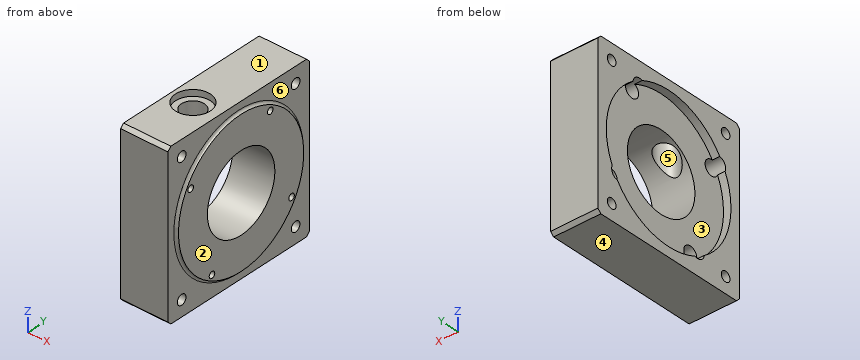
from build123d import *

# Parameters (mm, degrees)
SALIENTE_EXTRUIR1_DEPTH            = 38
TALADRO_DE_MARGEN_PARA_M1001_D     = 114.5
TALADRO_DE_MARGEN_PARA_M1001_DEPTH = 6
CROQUIS9_W                         = 34
CROQUIS9_H                         = 31
TALADRO_DE_MARGEN_PARA_M71_D       = 8


# Read off the part's stored shape, not the designer's step: Refrentado para perno con cabeza hexagonal de M161
with BuildPart() as part:
    # Croquis1 → Saliente-Extruir1 (new body)
    with BuildSketch(Plane(origin=(-94.5, 0, 0), x_dir=(0, -1, 0), z_dir=(-1, 0, 0))):
        with BuildLine():
            Line((62.24949799, 65), (-62.24949799, 65))
            ThreePointArc((-62.24949799, 65), (-63.639610307, 63.639610307), (-65, 62.24949799))
            Line((-65, 62.24949799), (-65, -62.24949799))
            ThreePointArc((-65, -62.24949799), (-63.639610307, -63.639610307), (-62.24949799, -65))
            Line((-62.24949799, -65), (62.24949799, -65))
            ThreePointArc((62.24949799, -65), (63.639610307, -63.639610307), (65, -62.24949799))
            Line((65, -62.24949799), (65, 62.24949799))
            ThreePointArc((65, 62.24949799), (63.639610307, 63.639610307), (62.24949799, 65))
        make_face()
    extrude(amount=-SALIENTE_EXTRUIR1_DEPTH)

    # Taladro de margen para M1001
    with Locations(Plane.ZY.offset(94.5)):
        with Locations((0, 0)):
            Hole(TALADRO_DE_MARGEN_PARA_M1001_D / 2, depth=TALADRO_DE_MARGEN_PARA_M1001_DEPTH)

    # Croquis4 → Revolución1 (revolve)
    with BuildSketch(Plane(origin=(0, 0, 0), x_dir=(-1, 0, 0), z_dir=(0, 0, -1)), mode=Mode.PRIVATE) as revoluci_n1_sk:
        with BuildLine():
            Line((54.5, 57.5), (54.5, 0))
            Line((54.5, 0), (56.5, 0))
            Line((56.5, 0), (56.5, 59.5))
            ThreePointArc((56.5, 59.5), (55.914213562, 58.085786438), (54.5, 57.5))
        make_face()
    revolve(revoluci_n1_sk.sketch.rotate(Axis((-54.499975, 0, 0), (-1, 0, 0)), 270), axis=Axis((-54.499975, 0, 0), (-1, 0, 0)))

    # Croquis5 → Cortar-Revolución1 (revolve, cut)
    with BuildSketch(Plane(origin=(0, 0, 46.3323591), x_dir=(-1, 0, 0), z_dir=(0, 0, -1)), mode=Mode.PRIVATE) as cortar_revoluci_n1_sk:
        Polygon((54.5, 29.3), (54.5, 26.75), (94.5, 26.75), (94.5, 32.75), (63.5, 32.75), (63.5, 29.3), align=None)
    revolve(cortar_revoluci_n1_sk.sketch.rotate(Axis((-54.5, 26.75, 46.3323591), (-1, 0, 0)), 270), axis=Axis((-54.5, 26.75, 46.3323591), (-1, 0, 0)), mode=Mode.SUBTRACT)

    # Croquis6 → Cortar-Revolución2 (revolve, cut)
    with BuildSketch(Plane(origin=(0, 0, -26.75), x_dir=(-1, 0, 0), z_dir=(0, 0, -1)), mode=Mode.PRIVATE) as cortar_revoluci_n2_sk:
        Polygon((54.5, 48.8823591), (54.5, 46.3323591), (94.5, 46.3323591), (94.5, 52.3323591), (63.5, 52.3323591), (63.5, 48.8823591), align=None)
    revolve(cortar_revoluci_n2_sk.sketch.rotate(Axis((-54.5, 46.3323591, -26.75), (-1, 0, 0)), 270), axis=Axis((-54.5, 46.3323591, -26.75), (-1, 0, 0)), mode=Mode.SUBTRACT)

    # Croquis7 → Cortar-Revolución3 (revolve, cut)
    with BuildSketch(Plane(origin=(0, 0, -46.3323591), x_dir=(-1, 0, 0), z_dir=(0, 0, -1)), mode=Mode.PRIVATE) as cortar_revoluci_n3_sk:
        Polygon((54.5, -24.2), (54.5, -26.75), (94.5, -26.75), (94.5, -20.75), (63.5, -20.75), (63.5, -24.2), align=None)
    revolve(cortar_revoluci_n3_sk.sketch.rotate(Axis((-54.5, -26.75, -46.3323591), (-1, 0, 0)), 270), axis=Axis((-54.5, -26.75, -46.3323591), (-1, 0, 0)), mode=Mode.SUBTRACT)

    # Croquis8 → Cortar-Revolución4 (revolve, cut)
    with BuildSketch(Plane(origin=(0, 0, 26.75), x_dir=(-1, 0, 0), z_dir=(0, 0, -1)), mode=Mode.PRIVATE) as cortar_revoluci_n4_sk:
        Polygon((54.5, -43.7823591), (54.5, -46.3323591), (94.5, -46.3323591), (94.5, -40.3323591), (63.5, -40.3323591), (63.5, -43.7823591), align=None)
    revolve(cortar_revoluci_n4_sk.sketch.rotate(Axis((-54.5, -46.3323591, 26.75), (-1, 0, 0)), 270), axis=Axis((-54.5, -46.3323591, 26.75), (-1, 0, 0)), mode=Mode.SUBTRACT)

    # Croquis9 → Cortar-Revolución5 (revolve, cut)
    with BuildSketch(Plane.XY, mode=Mode.PRIVATE) as cortar_revoluci_n5_sk:
        with Locations((-71.5, 15.5)):
            Rectangle(CROQUIS9_W, CROQUIS9_H)
    revolve(cortar_revoluci_n5_sk.sketch.rotate(Axis((-88.5, 0, 0), (1, 0, 0)), 270), axis=Axis((-88.5, 0, 0), (1, 0, 0)), mode=Mode.SUBTRACT)

    # Refrentado para perno con cabeza hex 2 → Refrentado para perno con cabeza hexagonal de M161 (revolve, cut)
    with BuildSketch(Plane(origin=(-77.5, -18, 0), x_dir=(1, 0, 0), z_dir=(0, -1, 0))):
        Polygon((0, 14.891701752), (9.188095, 14.891701752), (9.188095, 60), (14, 60), (14, 65), (0, 65), align=None)
    revolve(axis=Axis((-77.5, -18, 0), (0, 0, 1)), mode=Mode.SUBTRACT)

    # Taladro de margen para M71 (through all)
    with Locations(Plane.ZY.offset(94.5)):
        with Locations((-52.325901808, 52.325901808), (52.325901808, 52.325901808), (52.325901808, -52.325901808), (-52.325901808, -52.325901808)):
            Hole(TALADRO_DE_MARGEN_PARA_M71_D / 2)


solid = part.part
Verification items for the finished model (mm, model axes). Face numbers are marked on the shaded views. A direction names the side the tool comes from. Coordinates: 2 decimals unless noted, no trailing zeros. Order: outer loops, then holes, each group sorted by start corner. A loop starts at its lowest first (then second) coordinate and runs counter-clockwise, first axis right, second up. Notation, with made-up numbers: M 66.5,73 L 103.5,73 A26 ccw 103.5,91 Z; hole C -39,43 d2. An arc over 180 degrees is marked long. One line per item, written item: value. Start each with the question number.
Item 1: Depth check by flat-ended pin: P1, Ø6, axis at y = 22.5, z = 15, coming from the +X side; P2, Ø3.5, axis at y = -27, z = -44, coming from the -X side; P3, Ø9, axis at y = -52.33, z = 52.33, coming from the +X side; P4, Ø9.5, axis at y = -43.5, z = 26.5, coming from the -X side. Enter the tip coordinate at first touch or a pass-through.
Item 2: Sectioned sample at C-C on x = -77. Give the number of separate pieces and of enclosed holes in the cut face, then the cut area to 3 significant figures.
Item 3: Access from +Z, -Z, +X, -X, +Y, -Y to the whole of each face (thin tool, end or side, straight path). Record for the marked faces 4, 5 and 6.
Item 4: Sectioned sample at A-A on y = 0. Record the cut outline in (x, z).
Item 5: Thickness scan on probe 1 along Y at (x, z) = (-66, 52.5); probe 2 along Z at (x, y) = (-61, -26); probe 3 along Y at (x, z) = (-57.5, -26.75). Record the ranges inside material, lowest first.
Item 6: Mould release check, pull along Z, two halves, no side actions. Record for the marked faces 1, 2 and 3: pulls with the +Z half, pulls with the -Z half, needs draft (parallel to the pull), parting line crosses it, or undercut.
Calculated:
1. P1: through
1. P2: x = -63.5
1. P3: x = -56.5
1. P4: x = -88.5
2. separate pieces: 1
2. enclosed holes: 8
2. area: 12,400 mm^2
3. face 4: -Z, +X, -X, +Y, -Y
3. face 5: +Z
3. face 6: +X
4. outline: M -94.5,-65 L -56.5,-65 L -56.5,-59.5 A2 cw -54.5,-57.5 L -54.5,-31 L -88.5,-31 L -88.5,-57.25 L -94.5,-57.25 Z; M -94.5,57.25 L -88.5,57.25 L -88.5,31 L -54.5,31 L -54.5,57.5 A2 cw -56.5,59.5 L -56.5,65 L -94.5,65 Z
5. probe 1: -65 to -56.32, -48.33 to 48.33, 56.32 to 65
5. probe 2: -65 to -48.77, -43.9 to -16.88, 16.88 to 65
5. probe 3: -65 to -15.67, 15.67 to 43.78, 48.88 to 65
6. face 1: pulls with the +Z half
6. face 2: needs draft
6. face 3: undercut
